Here's how the part is built. I have some questions about the finished solid (model axes, mm). A direction names the side the tool comes from. Coordinates: 2 decimals unless noted, no trailing zeros. Order: outer loops, then holes, each group sorted by start corner. A loop starts at its lowest first (then second) coordinate and runs counter-clockwise, first axis right, second up. Notation, with made-up numbers: (-36.5, 34.25) -> (10.5, 34.25) arc R19 cw to (10.5, 62.25) -> close; hole circle Ø8 at (-1.75, 62.25). An arc over 180 degrees is marked (long way). One line per item, written item: value. Start each with the question number.
```python
from build123d import *

# Parameters (mm, degrees)
SKETCH1_W           = 36
SKETCH1_H           = 81
BOSS_EXTRUDE1_DEPTH = 11
SKETCH2_W           = 30
SKETCH2_H           = 75
CUT_EXTRUDE1_DEPTH  = 8
FILLET1_R           = 3
SKETCH3_W           = 1.6
SKETCH3_H           = 3
CUT_EXTRUDE2_DEPTH  = 0.8
SKETCH4_W           = 1
SKETCH4_H           = 5
SKETCH4_W_2         = 5
SKETCH4_H_2         = 1
CUT_EXTRUDE3_DEPTH  = 3


with BuildPart() as part:
    # Sketch1 → Boss-Extrude1 (new body)
    with BuildSketch(Plane(origin=(0, 0, 0), x_dir=(1, 0, 0), z_dir=(0, 1, 0))):
        with Locations((18, 40.5)):
            Rectangle(SKETCH1_W, SKETCH1_H)
    extrude(amount=BOSS_EXTRUDE1_DEPTH)

    # Sketch2 → Cut-Extrude1 (cut)
    with BuildSketch(Plane(origin=(0, 11, 0), x_dir=(1, 0, 0), z_dir=(0, 1, 0))):
        with Locations((18, 40.5)):
            Rectangle(SKETCH2_W, SKETCH2_H)
    extrude(amount=-CUT_EXTRUDE1_DEPTH, mode=Mode.SUBTRACT)

    # Fillet1
    fillet1_edges = [part.edges().sort_by_distance(p)[0] for p in [
        (0, 5.5, -81),
        (36, 5.5, -81),
        (36, 5.5, 0),
        (0, 5.5, 0),
    ]]
    fillet(fillet1_edges, radius=FILLET1_R)

    # Sketch3 → Cut-Extrude2 (cut)
    with BuildSketch(Plane(origin=(0, 11, 0), x_dir=(1, 0, 0), z_dir=(0, 1, 0))):
        with Locations((18, 79.5)):
            Rectangle(SKETCH3_W, SKETCH3_H)
    extrude(amount=-CUT_EXTRUDE2_DEPTH, mode=Mode.SUBTRACT)

    # Sketch4 → Cut-Extrude3 (cut)
    with BuildSketch(Plane(origin=(0, 11, 0), x_dir=(1, 0, 0), z_dir=(0, 1, 0))):
        with Locations((2.5, 40.5)):
            Rectangle(SKETCH4_W, SKETCH4_H)
        with Locations((33.5, 40.5)):
            Rectangle(SKETCH4_W, SKETCH4_H)
        with Locations((18, 2.5)):
            Rectangle(SKETCH4_W_2, SKETCH4_H_2)
    extrude(amount=-CUT_EXTRUDE3_DEPTH, mode=Mode.SUBTRACT)


solid = part.part
```
Q1. For P1, Ø15, axis at x = 22, z = -51.5, coming from the +Y side; P2, Ø0.5, axis at x = 33.5, z = -39.5, coming from the +Y side; P3, Ø0.8, axis at x = 18, z = -80, coming from the +Y side, each with a flat end and sliding along its axis, tell me the tip position at first contact or that it passes through.
Q2. For faces 1 (the face through (18, 10.2, -80)), 2 (the face through (18, 10, -2)), 3 (the face through (35.1, 5.58, -80.14)), which set-ups out of +Z, -Z, +X, -X, +Y, -Y let a thin tool reach every point of the face, with its end or its side?
Q3. Imagine slicing it at B-B (x = 31.5). Write out the boundary of the cut face in (y, z).
Q4. I need wall thicknesses on line 1 (X direction, y = 4.75, z = -21); line 2 (Z direction, x = 30, y = 3.25); line 3 (Y direction, x = 9, z = -44.5). Which ranges of each line are inside material? Lowest first, please.
Q5. Imagine slicing it at A-A (y = 6.75). Write out the boundary of the cut face in (x, z).
Q6. Imagine slicing it at C-C (z = -13). Write out the boundary of the cut face in (x, y).
Q7. If we mould it in two halves opening along X, with no side actions, what happens to faces 4 (the face through (18, 5, -81)), 5 (the face through (0, 5, -40)), 6 (the face through (18, 3, -41))? For each: +X half, -X half, draft (parallel to the pull), parting line (faces both ways), or undercut.
Completed:
1. P1: stops at y = 3
1. P2: stops at y = 8
1. P3: stops at y = 10.2
2. face 1: -Z, +Y
2. face 2: +Y
2. face 3: -Z, +X, +Y, -Y
3. outline: (0, -81) -> (11, -81) -> (11, -78) -> (3, -78) -> (3, -3) -> (11, -3) -> (11, 0) -> (0, 0) -> close
4. line 1: x = 0 to 3, 33 to 36
4. line 2: z = -81 to -78, -3 to 0
4. line 3: y = 0 to 3
5. outline: (0, -78) arc R3 ccw to (3, -81) -> (33, -81) arc R3 ccw to (36, -78) -> (36, -3) arc R3 ccw to (33, 0) -> (3, 0) arc R3 ccw to (0, -3) -> close; hole (3, -78) -> (33, -78) -> (33, -3) -> (3, -3) -> close
6. outline: (0, 0) -> (36, 0) -> (36, 11) -> (33, 11) -> (33, 3) -> (3, 3) -> (3, 11) -> (0, 11) -> close
7. face 4: draft
7. face 5: -X half
7. face 6: undercut
